For this review, take the finished solid that the model builds, in its own axes (mm). A direction names the side the tool comes from. Round coordinates to 2 decimals unless told otherwise and drop trailing zeros. Loops run counter-clockwise (first coordinate to the right, second up) from the corner with the lowest first, then second, coordinate; pieces in that order, holes last.
1. Consider section D-D on x = -11. State the section outline as (y, z) points.
2. Clearance check with flat-ended pins moving along their axes: pin 1 Ø5 at (x, y) = (1, 4) entering from +Z; pin 2 Ø3 at (x, y) = (9.5, -13.5) entering from -Z; pin 3 Ø3 at (x, z) = (-14, -1) entering from -Y; pin 4 Ø6.5 at (x, y) = (-12.5, 0.5) entering from +Z. State where each tip first meets the part, or that it passes through.
3. Draft analysis for pull direction Y (two halves, no side actions). For faces 1 (the flat face through (-4, 2, 3)), 2 (the flat face through (9, 0, -12)), state which applies: released by +Y, released by -Y, zero draft, split by the parting line, or undercut.
4. Consider section B-B on z = 6. State the section outline as (x, y) points.
5. Tool access review of faces 3 (the cylindrical face through (-12.354, 0.676, 1.977)), 4 (the flat face through (-4, -2, -7)), 5 (the cylindrical face through (-0.521, 18.466, 5.979)): name each direction out of +Z, -Z, +X, -X, +Y, -Y from which nothing blocks a thin tool from reaching the whole face with its end or side.
6. To check wall thickness, follow line 1 along Y through (x, z) = (0, 6); line 2 along Z through (x, y) = (14, 13); line 3 along X through (y, z) = (-1.5, -6.25). State the ranges of each line that lie inside material, in increasing order.
7. Consider section A-A on y = -13.5. State the section outline as (x, z) points.
from build123d import *
from build123d.topology import SkipClean

# Parameters (mm, degrees)
SKETCH_1_R           = 19.5
EXTRUDE_1_DEPTH      = 6
SKETCH_2_R           = 9.5
EXTRUDE_2_DEPTH      = 3
SKETCH_3_R           = 5
CUT_EXTRUDE_1_DEPTH  = 50
SKETCH_4_R           = 4
CUT_EXTRUDE_2_DEPTH  = 4.4
SKETCH_5_R           = 2.25
CUT_EXTRUDE_3_DEPTH  = 4.4
SKETCH_6_R           = 2.25
CUT_EXTRUDE_4_DEPTH  = 4.4
SKETCH_7_R           = 2.25
CUT_EXTRUDE_5_DEPTH  = 4.4
SKETCH_8_R           = 10.5
EXTRUDE_3_DEPTH      = 12
SKETCH_9_R           = 8.5
CUT_EXTRUDE_6_DEPTH  = 20
SKETCH_10_R          = 19.5
EXTRUDE_4_DEPTH      = 8
CUT_EXTRUDE_START    = -8
SKETCH_11_R          = 8.5
CUT_EXTRUDE_8_DEPTH  = 8
SKETCH_12_R          = 4
CUT_EXTRUDE_10_DEPTH = 4.1
SKETCH_13_R          = 2.25
CUT_EXTRUDE_11_DEPTH = 4.1
EXTRUDE_START        = -20
SKETCH_14_R          = 8.5
EXTRUDE_5_DEPTH      = 20
SKETCH_15_R          = 8.5
CUT_EXTRUDE_12_DEPTH = 5
SKETCH_17_R          = 4
EXTRUDE_7_DEPTH      = 2.35
SKETCH_18_R          = 3
CUT_EXTRUDE_13_DEPTH = 20
CUT_EXTRUDE_START_2  = -5
SKETCH_19_R          = 8.5
CUT_EXTRUDE_14_DEPTH = 5
EXTRUDE_START_2      = 2.35
SKETCH_20_R          = 4
EXTRUDE_8_DEPTH      = 2.35
CUT_EXTRUDE_START_3  = -2.35
SKETCH_21_R          = 3
CUT_EXTRUDE_15_DEPTH = 2.35


with BuildPart() as part:
    # 草图1 → 凸台-拉伸1 (new body)
    with BuildSketch(Plane.XY):
        Circle(SKETCH_1_R)
    extrude(amount=EXTRUDE_1_DEPTH)

    # 草图2 → 凸台-拉伸2 (add)
    with BuildSketch(Plane(origin=(0, 0, 0), x_dir=(-1, 0, 0), z_dir=(0, 0, -1))):
        Circle(SKETCH_2_R)
    extrude(amount=EXTRUDE_2_DEPTH)

    # 草图3 → 切除-拉伸1 (cut)
    with BuildSketch(Plane(origin=(0, 0, -3), x_dir=(-1, 0, 0), z_dir=(0, 0, -1))):
        Circle(SKETCH_3_R)
    extrude(amount=-CUT_EXTRUDE_1_DEPTH, mode=Mode.SUBTRACT)

    # 草图4 → 切除-拉伸2 (cut)
    with BuildSketch(Plane.XY.offset(6)):
        with Locations((0, 14.5)):
            Circle(SKETCH_4_R)
        with Locations((14.5, 0)):
            Circle(SKETCH_4_R)
        with Locations((0, -14.5)):
            Circle(SKETCH_4_R)
        with Locations((-14.5, 0)):
            Circle(SKETCH_4_R)
    extrude(amount=-CUT_EXTRUDE_2_DEPTH, mode=Mode.SUBTRACT)

    # 草图5 → 切除-拉伸3 (cut)
    with BuildSketch(Plane.XY.offset(1.6)):
        with Locations((-14.5, 0)):
            Circle(SKETCH_5_R)
    extrude(amount=-CUT_EXTRUDE_3_DEPTH, mode=Mode.SUBTRACT)

    # 草图6 → 切除-拉伸4 (cut)
    with BuildSketch(Plane.XY.offset(1.6)):
        with Locations((0, 14.5)):
            Circle(SKETCH_6_R)
    extrude(amount=-CUT_EXTRUDE_4_DEPTH, mode=Mode.SUBTRACT)

    # 草图7 → 切除-拉伸5 (cut)
    with BuildSketch(Plane.XY.offset(1.6)):
        with Locations((14.5, 0)):
            Circle(SKETCH_7_R)
        with Locations((0, -14.5)):
            Circle(SKETCH_7_R)
    extrude(amount=-CUT_EXTRUDE_5_DEPTH, mode=Mode.SUBTRACT)

    # 草图8 → 凸台-拉伸3 (add)
    with BuildSketch(Plane(origin=(0, 0, 0), x_dir=(-1, 0, 0), z_dir=(0, 0, -1))):
        with Locations(Location((0, 0, 0), (0, 0, 180))):
            Circle(SKETCH_8_R)
    extrude(amount=EXTRUDE_3_DEPTH)

    # 草图9 → 切除-拉伸6 (cut)
    with BuildSketch(Plane(origin=(0, 0, -12), x_dir=(-1, 0, 0), z_dir=(0, 0, -1))):
        Circle(SKETCH_9_R)
    extrude(amount=-CUT_EXTRUDE_6_DEPTH, mode=Mode.SUBTRACT)

    # 草图10 → 凸台-拉伸4 (add)
    with SkipClean():  # the faces are left unmerged after this step: merging them gives an invalid solid
        with BuildSketch(Plane(origin=(0, 0, 0), x_dir=(-1, 0, 0), z_dir=(0, 0, -1))):
            Circle(SKETCH_10_R)
        extrude(amount=-EXTRUDE_4_DEPTH)

    # 草图11 → 切除-拉伸8 (cut)
    with SkipClean():  # the faces are left unmerged after this step: merging them gives an invalid solid
        with BuildSketch(Plane.XY.offset(8).offset(CUT_EXTRUDE_START)):
            with Locations(Location((0, 0, 0), (0, 0, 180))):
                Circle(SKETCH_11_R)
        extrude(amount=CUT_EXTRUDE_8_DEPTH, mode=Mode.SUBTRACT)

    # 草图12 → 切除-拉伸10 (cut)
    with SkipClean():  # the faces are left unmerged after this step: merging them gives an invalid solid
        with BuildSketch(Plane.XY.offset(8)):
            with Locations((0, 14.5)):
                Circle(SKETCH_12_R)
            with Locations((14.5, 0)):
                Circle(SKETCH_12_R)
            with Locations((0, -14.5)):
                Circle(SKETCH_12_R)
            with Locations((-14.5, 0)):
                Circle(SKETCH_12_R)
        extrude(amount=-CUT_EXTRUDE_10_DEPTH, mode=Mode.SUBTRACT)

    # 草图13 → 切除-拉伸11 (cut)
    with SkipClean():  # the faces are left unmerged after this step: merging them gives an invalid solid
        with BuildSketch(Plane.XY.offset(3.9)):
            with Locations((0, 14.5)):
                Circle(SKETCH_13_R)
            with Locations((14.5, 0)):
                Circle(SKETCH_13_R)
            with Locations((0, -14.5)):
                Circle(SKETCH_13_R)
            with Locations((-14.5, 0)):
                Circle(SKETCH_13_R)
        extrude(amount=-CUT_EXTRUDE_11_DEPTH, mode=Mode.SUBTRACT)

    # 草图14 → 凸台-拉伸5 (add)
    with SkipClean():  # the faces are left unmerged after this step: merging them gives an invalid solid
        with BuildSketch(Plane.XY.offset(8).offset(EXTRUDE_START)):
            Circle(SKETCH_14_R)
        extrude(amount=EXTRUDE_5_DEPTH)

    # 草图15 → 切除-拉伸12 (cut)
    with SkipClean():  # the faces are left unmerged after this step: merging them gives an invalid solid
        with BuildSketch(Plane(origin=(0, 0, -12), x_dir=(-1, 0, 0), z_dir=(0, 0, -1))):
            Circle(SKETCH_15_R)
        extrude(amount=-CUT_EXTRUDE_12_DEPTH, mode=Mode.SUBTRACT)

    # 草图17 → 凸台-拉伸7 (add)
    with SkipClean():  # the faces are left unmerged after this step: merging them gives an invalid solid
        with BuildSketch(Plane(origin=(0, 0, -7), x_dir=(-1, 0, 0), z_dir=(0, 0, -1))):
            Circle(SKETCH_17_R)
        extrude(amount=EXTRUDE_7_DEPTH)

    # 草图18 → 切除-拉伸13 (cut)
    with SkipClean():  # the faces are left unmerged after this step: merging them gives an invalid solid
        with BuildSketch(Plane(origin=(0, 0, -9.35), x_dir=(-1, 0, 0), z_dir=(0, 0, -1))):
            Circle(SKETCH_18_R)
        extrude(amount=-CUT_EXTRUDE_13_DEPTH, mode=Mode.SUBTRACT)

    # 草图19 → 切除-拉伸14 (cut)
    with SkipClean():  # the faces are left unmerged after this step: merging them gives an invalid solid
        with BuildSketch(Plane.XY.offset(8).offset(CUT_EXTRUDE_START_2)):
            with Locations(Location((0, 0, 0), (0, 0, 180))):
                Circle(SKETCH_19_R)
        extrude(amount=CUT_EXTRUDE_14_DEPTH, mode=Mode.SUBTRACT)

    # 草图20 → 凸台-拉伸8 (add)
    with SkipClean():  # the faces are left unmerged after this step: merging them gives an invalid solid
        with BuildSketch(Plane.XY.offset(3).offset(EXTRUDE_START_2)):
            with Locations(Location((0, 0, 0), (0, 0, 180))):
                Circle(SKETCH_20_R)
        extrude(amount=-EXTRUDE_8_DEPTH)

    # 草图21 → 切除-拉伸15 (cut)
    with SkipClean():  # the faces are left unmerged after this step: merging them gives an invalid solid
        with BuildSketch(Plane.XY.offset(5.35).offset(CUT_EXTRUDE_START_3)):
            with Locations(Location((0, 0, 0), (0, 0, 180))):
                Circle(SKETCH_21_R)
        extrude(amount=CUT_EXTRUDE_15_DEPTH, mode=Mode.SUBTRACT)


solid = part.part
Resolved:
1. outline: (-16.1, 0) - (16.1, 0) - (16.1, 8) - (1.94, 8) - (1.94, 3.9) - (-1.94, 3.9) - (-1.94, 8) - (-16.1, 8) - close
2. pin 1: stops at z = 5.35
2. pin 2: stops at z = 0
2. pin 3: stops at y = -14.64
2. pin 4: stops at z = 8
3. face 1: undercut
3. face 2: zero draft
4. outline: circle Ø39 at (0, 0); hole circle Ø8 at (-14.5, 0); hole circle Ø17 at (0, 0); hole circle Ø8 at (0, -14.5); hole circle Ø8 at (0, 14.5); hole circle Ø8 at (14.5, 0)
5. face 3: +Z, -Z
5. face 4: -Z
5. face 5: +Z
6. line 1: y = -19.5 to -18.5, -10.5 to -8.5, 8.5 to 10.5, 18.5 to 19.5
6. line 2: z = 0 to 8
6. line 3: x = -10.39 to -2.6, 2.6 to 10.39
7. outline: (-14.07, 0) - (-2.02, 0) - (-2.02, 3.9) - (-3.87, 3.9) - (-3.87, 8) - (-14.07, 8) - close; (2.02, 0) - (14.07, 0) - (14.07, 8) - (3.87, 8) - (3.87, 3.9) - (2.02, 3.9) - close
